Model file for the job. Use its own axes, mm. Face numbers are marked on the shaded views. A direction names the side the tool comes from. Round coordinates to 2 decimals unless told otherwise and drop trailing zeros. Loops run counter-clockwise (first coordinate to the right, second up) from the corner with the lowest first, then second, coordinate; pieces in that order, holes last. Notation, with made-up numbers: M 37.5,-26 L 50.5,-26 A37 ccw 50.5,13 Z; hole C -8,56 d2. An arc over 180 degrees is marked long. Answer in a Markdown table with one row per item.
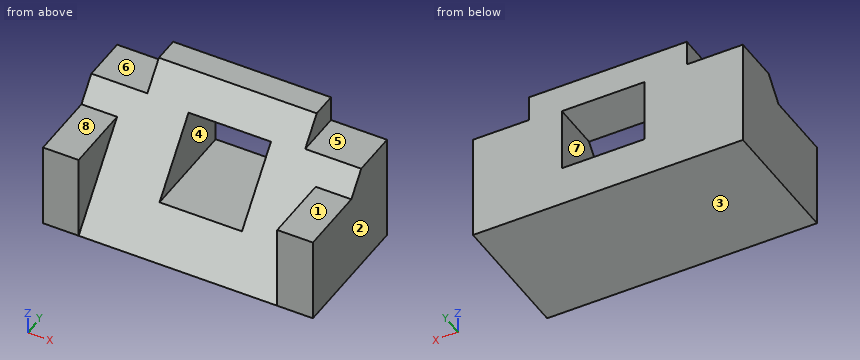
from build123d import *

# Parameters (mm, degrees)
PAD_DEPTH       = 26.5
PAD_DEPTH_BACK  = 26.5
SKETCH001_W     = 5
SKETCH001_H     = 11
POCKET_DEPTH    = 155.012627
SKETCH002_W     = 16.7
SKETCH002_H     = 7
PAD001_DEPTH    = 26
SKETCH004_W     = 12.588901
SKETCH004_H     = 16.182331
POCKET001_DEPTH = 26.001


with BuildPart() as part:
    # Sketch → Pad (new body, two sides)
    with BuildSketch(Plane.YZ) as pad_sk:
        Polygon((-26, 0), (-5, 26), (0, 26), (0, 0), align=None)
    extrude(amount=PAD_DEPTH)
    extrude(pad_sk.sketch, amount=-PAD_DEPTH_BACK)

    # Sketch001 (on Face3 of Pad) → Pocket (cut, through all)
    with BuildSketch(Plane.ZX):
        with Locations((23.5, 21)):
            Rectangle(SKETCH001_W, SKETCH001_H)
    pocket = extrude(amount=-POCKET_DEPTH, mode=Mode.SUBTRACT)

    # Mirrored: Pocket across Sketch001 H_Axis
    add(pocket.mirror(Plane.YZ), mode=Mode.SUBTRACT)

    # Sketch002 (on Face10 of Mirrored) → Pad001 (join)
    with BuildSketch(Plane.ZX):
        with Locations((8.35, 23)):
            Rectangle(SKETCH002_W, SKETCH002_H)
    pad001 = extrude(amount=-PAD001_DEPTH)

    # Mirrored001: Pad001 across Sketch002 H_Axis
    add(pad001.mirror(Plane.YZ))

    # Sketch004 (on Face6 of Mirrored001) → Pocket001 (cut, through all)
    with BuildSketch(Plane.ZX):
        with Locations((14.102484, 0.951072)):
            Rectangle(SKETCH004_W, SKETCH004_H)
    extrude(amount=-POCKET001_DEPTH, mode=Mode.SUBTRACT)


solid = part.part
1. Pin check, flat tips, straight feed: pin 1 (3 mm diameter, centred on x = 13.5, y = -11, fed in from +Z); pin 2 (5.5 mm diameter, centred on y = -4, z = 24, fed in from -X); pin 3 (5.5 mm diameter, centred on x = 22.5, y = -22, fed in from +Z). Stop position of each tip, or through.
Verdict:
| item | result |
|---|---|
| pin 1 | stops at z = 20.43 |
| pin 2 | stops at x = -15.5 |
| pin 3 | stops at z = 16.7 |
2. Wall check: probe 1 along X at (y, z) = (-17.75, 8); probe 2 along Z at (x, y) = (-18, -4.25); probe 3 along X at (y, z) = (-3, 22.25). Give the ranges that are in metal, low to high.
Verdict:
| item | result |
|---|---|
| probe 1 | x = -26.5 to -7.14, 9.04 to 26.5 |
| probe 2 | z = 0 to 21 |
| probe 3 | x = -15.5 to 15.5 |
3. Mould opens along Z. For the marked faces 1, 2, 3 and 4 say: +Z half, -Z half, draft (parallel to the pull), parting line (faces both ways), or undercut.
Verdict:
| item | result |
|---|---|
| face 1 | +Z half |
| face 2 | draft |
| face 3 | -Z half |
| face 4 | undercut |
4. Saw through at C-C (z = 10.75). Write the cut outline in (x, y).
Verdict:
| item | result |
|---|---|
| outline | M -26.5,-26 L -19.5,-26 L -19.5,-17.32 L -7.14,-17.32 L -7.14,0 L -26.5,0 Z; M 9.04,-17.32 L 19.5,-17.32 L 19.5,-26 L 26.5,-26 L 26.5,0 L 9.04,0 Z |
5. Saw through at D-D (y = -24.25). Write the cut outline in (x, z).
Verdict:
| item | result |
|---|---|
| outline | M -26.5,0 L 26.5,0 L 26.5,16.7 L 19.5,16.7 L 19.5,2.17 L -19.5,2.17 L -19.5,16.7 L -26.5,16.7 Z |
6. Saw through at A-A (x = 2.5). Write the cut outline in (y, z), and give its area (3 significant figures).
Verdict:
| item | result |
|---|---|
| outline | M -26,0 L 0,0 L 0,7.81 L -19.69,7.81 Z; M -9.53,20.4 L 0,20.4 L 0,26 L -5,26 Z |
| area | 219 mm² |
7. Tool access for the marked faces 5, 6, 7 and 8: list every direction of +Z, -Z, +X, -X, +Y, -Y with a clear straight run to the whole face (end or side of a thin tool).
Verdict:
| item | result |
|---|---|
| face 5 | +Z, +X, +Y, -Y |
| face 6 | +Z, -X, +Y, -Y |
| face 7 | +Y, -Y |
| face 8 | +Z, +X, -X, -Y |
8. Saw through at B-B (y = -4.25). Write the cut outline in (x, z), and give its area (3 significant figures).
Verdict:
| item | result |
|---|---|
| outline | M -26.5,0 L 26.5,0 L 26.5,21 L 15.5,21 L 15.5,26 L -15.5,26 L -15.5,21 L -26.5,21 Z; hole M -7.14,7.81 L 9.04,7.81 L 9.04,20.4 L -7.14,20.4 Z |
| area | 1,060 mm² |
